The listing builds one solid part. Answer for the finished solid, in the listing's coordinates (mm). A direction names the side the tool comes from. Round coordinates to 2 decimals unless told otherwise and drop trailing zeros. Loops run counter-clockwise (first coordinate to the right, second up) from the corner with the lowest first, then second, coordinate; pieces in that order, holes last. Notation, with made-up numbers: (30, 17.5) - (34, 17.5) arc R19 cw to (34, 52.5) - close; hole circle Ø2 at (5, 69). An arc over 180 degrees is marked (long way). One line per question, with ' | ' between items. Start each with the question number.
from build123d import *

# Parameters (mm, degrees)
F0_R     = 34
F1_DEPTH = 6
F2_W     = 4.1
F2_H     = 2.7
F4_R     = 5
F5_DEPTH = 2


with BuildPart() as f1:
    # F0 (on Top) → F1 (new body)
    with BuildSketch(Plane.XY):
        Circle(F0_R)
    extrude(amount=F1_DEPTH)

    # F2 (on Right) → F3 (revolve, cut)
    with BuildSketch(Plane.YZ):
        with Locations((2.05, 1.35)):
            Rectangle(F2_W, F2_H)
    revolve(axis=Axis((0, 0, 1.35), (0, 0, -1)), mode=Mode.SUBTRACT)

    # F4 (on face) → F5 (cut)
    with BuildSketch(Plane(origin=(0, 0, 2.7), x_dir=(1, 0, 0), z_dir=(0, 0, -1))):
        Circle(F4_R)
    extrude(amount=-F5_DEPTH, mode=Mode.SUBTRACT)


solid = f1.part
(1) Each of these flat-tipped pins is pushed along its axis until it touches: P1, Ø9, axis at x = 0, y = 0, coming from the -Z side; P2, Ø7.5, axis at x = 0, y = 0, coming from the -Z side; P3, Ø1, axis at y = 18.5, z = 4.5, coming from the -X side; P4, Ø1, axis at x = 24, z = 5.5, coming from the +Y side. Where does it stop, or does it pass through?
(2) Determine the mould class of faces 4 (the flat face through (-4, -2, 2.7)), 5 (the cylindrical face through (18.28, 28.67, 2.96)), 6 (the flat face through (0, 0, 6)) for opening direction Z: pulls with the +Z half, pulls with the -Z half, needs draft (parallel to the pull), parting line crosses it, or undercut.
(3) Find section C-C on x = 3. Write down the section's boundary in (y, z), plus the area to 3 significant figures.
(4) A tool of negligible diameter and unlimited length cuts with its end or side. For faces 1 (the cylindrical face through (-1.08, 4.88, 3.69)), 2 (the cylindrical face through (4.065, -0.534, 1.369)), 3 (the flat face through (7, 0, 0)), from which of +Z, -Z, +X, -X, +Y, -Y can it reach the whole face along a straight path? Write none if from no direction.
(5) Find section A-A on y = 0. Write down the section's boundary in (x, z), plus the area to 3 significant figures.
(6) Find section B-B on z = 0.95. Write down the section's boundary in (x, y), plus the area to 3 significant figures.
(7) Find section D-D on y = 27. Write down the section's boundary in (x, z).
(8) Consider L1, parallel to Y at x = 0, z = 3.25; L2, parallel to X at y = 17.5, z = 2.6; L3, parallel to X at y = -25, z = 1.4. Determine where each line is inside the solid, lowest interval first.
Answer below:
1) P1: z = 0 | P2: z = 4.7 | P3: x = -28.84 | P4: y = 24.57
2) face 4: undercut | face 5: needs draft | face 6: pulls with the +Z half
3) outline: (-33.87, 0) - (-2.79, 0) - (-2.79, 2.7) - (-4, 2.7) - (-4, 4.7) - (4, 4.7) - (4, 2.7) - (2.79, 2.7) - (2.79, 0) - (33.87, 0) - (33.87, 6) - (-33.87, 6) - close | area: 375 mm2
4) face 1: none | face 2: -Z | face 3: -Z, +X, -X, +Y, -Y
5) outline: (-34, 0) - (-4.1, 0) - (-4.1, 2.7) - (-5, 2.7) - (-5, 4.7) - (5, 4.7) - (5, 2.7) - (4.1, 2.7) - (4.1, 0) - (34, 0) - (34, 6) - (-34, 6) - close | area: 366 mm2
6) outline: circle Ø68 at (0, 0); hole circle Ø8.2 at (0, 0) | area: 3,580 mm2
7) outline: (-20.66, 0) - (20.66, 0) - (20.66, 6) - (-20.66, 6) - close
8) L1: -34 to -5, 5 to 34 | L2: -29.15 to 29.15 | L3: -23.04 to 23.04
